Read the model definition and answer for the solid it produces. Units are mm, in the model's axes. A direction names the side the tool comes from. Round coordinates to 2 decimals unless told otherwise and drop trailing zeros. Order: outer loops, then holes, each group sorted by start corner. A loop starts at its lowest first (then second) coordinate and runs counter-clockwise, first axis right, second up. Notation, with made-up numbers: (13.25, 3) -> (68.25, 3) arc R15 cw to (68.25, 25) -> close; hole circle Ø6 at (62, 63.25). An arc over 180 degrees is marked (long way). Use a Markdown table: item, result. Add a question column.
1. Given pin 1 (2 mm diameter, centred on y = 22, z = 7.5, fed in from +X); pin 2 (8 mm diameter, centred on y = 42.5, z = 12.5, fed in from -X); pin 3 (13 mm diameter, centred on x = -28, z = -2.5, fed in from -Y); pin 4 (12 mm diameter, centred on x = 41.5, y = 20, fed in from -Z), each flat-ended and moving along its own axis, determine where each tip first touches the part or whether it passes through.
2. Consider L1, parallel to Z at x = 68.5, y = 6; L2, parallel to Z at x = 45.5, y = 16; L3, parallel to X at y = 5.5, z = 0.25. Determine where each line is inside the solid, lowest interval first. Write a range as [from, to].
3. For faces 1 (the face through (0, 82, -8)), 2 (the face through (-64.177, 47.376, 0.112)), determine the directions among +Z, -Z, +X, -X, +Y, -Y from which every point of the face is accessible in a straight line to the end or side of a thin tool.
4. The mould has two halves that part along X. Classify faces 3 (the face through (63.2, 16.13, 15.15)), 4 (the face through (-63.59, 81.62, -0.11)), 5 (the face through (-68.17, 4.69, -5)), 6 (the face through (-60.88, 78.68, 0.11)): +X half, -X half, draft (parallel to the pull), parting line (faces both ways), or undercut.
5. Section B-B, the plane y = 6 is taken. Give the vertices of the cut face in (x, z), then the cut area to 3 significant figures.
6. Section D-D, the plane z = -4 is taken. Give the number of separate pieces and of enclosed holes in the cut face, then the cut area to 3 significant figures.
7. Section C-C, the plane y = 32.5 is taken. Give the vertices of the cut face in (x, z).
8. Section A-A, the plane x = 54 is taken. Give the vertices of the cut face in (y, z), then the cut area to 3 significant figures.
```python
from build123d import *

# Parameters (mm, degrees)
PAD_DEPTH         = 8
SKETCH001_R       = 1.65
POCKET_DEPTH      = 70.201
POCKET_DEPTH_BACK = -70.201
FILLET001_R       = 9
FILLET002_R       = 5
FILLET003_R       = 2
FILLET004_R       = 1.99
PAD001_DEPTH      = 4
FILLET005_R       = 1.99
FILLET006_R       = 2
FILLET007_R       = 9.99


with BuildPart() as part:
    # Sketch → Pad (new body, symmetric)
    with BuildSketch(Plane.XY):
        Polygon((-70.2, 0), (-66.2, 0), (-66.2, 14), (-62.2, 80), (62.2, 80), (66.2, 14), (66.2, 0), (70.2, 0), (70.2, 14.121101), (65.964915, 84), (-65.964915, 84), (-70.2, 14.121101), align=None)
    extrude(amount=PAD_DEPTH, both=True)

    # Sketch001 → Pocket (cut, two sides)
    with BuildSketch(Plane.YZ) as pocket_sk:
        with Locations((6, 4)):
            Circle(SKETCH001_R)
        with Locations((6, -4)):
            Circle(SKETCH001_R)
    extrude(amount=-POCKET_DEPTH, mode=Mode.SUBTRACT)
    extrude(pocket_sk.sketch, amount=-POCKET_DEPTH_BACK, mode=Mode.SUBTRACT)

    # Fillet001
    fillet001_edges = [part.edges().sort_by_distance(p)[0] for p in [
        (-65.964915, 84, 0),
        (65.964915, 84, 0),
    ]]
    fillet(fillet001_edges, radius=FILLET001_R)

    # Fillet002
    fillet002_edges = [part.edges().sort_by_distance(p)[0] for p in [
        (62.2, 80, 0),
        (-62.2, 80, 0),
    ]]
    fillet(fillet002_edges, radius=FILLET002_R)

    # Fillet003
    fillet003_edges = [part.edges().sort_by_distance(p)[0] for p in [
        (-70.2, 0, 0),
        (70.2, 0, 0),
    ]]
    fillet(fillet003_edges, radius=FILLET003_R)

    # Fillet004
    fillet004_edges = [part.edges().sort_by_distance(p)[0] for p in [
        (-66.2, 0, 0),
        (66.2, 0, 0),
    ]]
    fillet(fillet004_edges, radius=FILLET004_R)

    # Sketch002 (on DatumPlane) → Pad001 (join)
    with BuildSketch(Plane.XZ.offset(-14.1)):
        Polygon((-58.7, -8), (-66.2, -8), (-66.2, 18), (66.2, 18), (66.2, -8), (58.7, -8), (58.7, 8), (-58.7, 8), align=None)
    extrude(amount=-PAD001_DEPTH)

    # Fillet005
    fillet005_edges = [part.edges().sort_by_distance(p)[0] for p in [
        (-58.7, 14.1, 0),
        (58.7, 14.1, 0),
    ]]
    fillet(fillet005_edges, radius=FILLET005_R)

    # Fillet006
    fillet006_edges = [part.edges().sort_by_distance(p)[0] for p in [
        (-65.951515, 18.1, 0),
        (-58.7, 18.1, 0),
        (58.7, 18.1, 0),
        (65.951515, 18.1, 0),
    ]]
    fillet(fillet006_edges, radius=FILLET006_R)

    # Fillet007
    fillet007_edges = [part.edges().sort_by_distance(p)[0] for p in [
        (66.2, 16.1, 18),
        (-66.2, 16.1, 18),
    ]]
    fillet(fillet007_edges, radius=FILLET007_R)


solid = part.part
```
Verdict:
| question | item | result |
|---|---|---|
| 1 | pin 1 | stops at x = 69.78 |
| 1 | pin 2 | passes through |
| 1 | pin 3 | stops at y = 80 |
| 1 | pin 4 | stops at z = 8 |
| 2 | L1 | z = [-8, -5.65], [-2.35, 2.35], [5.65, 8] |
| 2 | L2 | z = [8, 18] |
| 2 | L3 | x = [-70.2, -66.2], [66.2, 70.2] |
| 3 | face 1 | -Z, +X, -X, +Y, -Y |
| 3 | face 2 | +Z, -Z |
| 4 | face 3 | +X half |
| 4 | face 4 | -X half |
| 4 | face 5 | draft |
| 4 | face 6 | undercut |
| 5 | outline | (-70.2, -8) -> (-66.2, -8) -> (-66.2, -5.65) -> (-70.2, -5.65) -> close; (-70.2, -2.35) -> (-66.2, -2.35) -> (-66.2, 2.35) -> (-70.2, 2.35) -> close; (-70.2, 5.65) -> (-66.2, 5.65) -> (-66.2, 8) -> (-70.2, 8) -> close; (66.2, -8) -> (70.2, -8) -> (70.2, -5.65) -> (66.2, -5.65) -> close; (66.2, -2.35) -> (70.2, -2.35) -> (70.2, 2.35) -> (66.2, 2.35) -> close; (66.2, 5.65) -> (70.2, 5.65) -> (70.2, 8) -> (66.2, 8) -> close |
| 5 | area | 75.2 mm2 |
| 6 | separate pieces | 3 |
| 6 | enclosed holes | 0 |
| 6 | area | 1,180 mm2 |
| 7 | outline | (-69.09, -8) -> (-65.08, -8) -> (-65.08, 8) -> (-69.09, 8) -> close; (65.08, -8) -> (69.09, -8) -> (69.09, 8) -> (65.08, 8) -> close |
| 8 | outline | (14.1, 8) -> (18.1, 8) -> (18.1, 18) -> (14.1, 18) -> close; (80, -8) -> (84, -8) -> (84, 8) -> (80, 8) -> close |
| 8 | area | 104 mm2 |
